Verification items for the finished model (mm, model axes). Face numbers are marked on the shaded views. A direction names the side the tool comes from. Round coordinates to 2 decimals unless told otherwise and drop trailing zeros. Loops run counter-clockwise (first coordinate to the right, second up) from the corner with the lowest first, then second, coordinate; pieces in that order, holes last. Notation, with made-up numbers: (2.5, 16) - (53.5, 16) arc R27 ccw to (53.5, 34) - close; hole circle Ø7 at (50, 45). An arc over 180 degrees is marked (long way). Use CSV: the item, a comma, the result in double quotes.
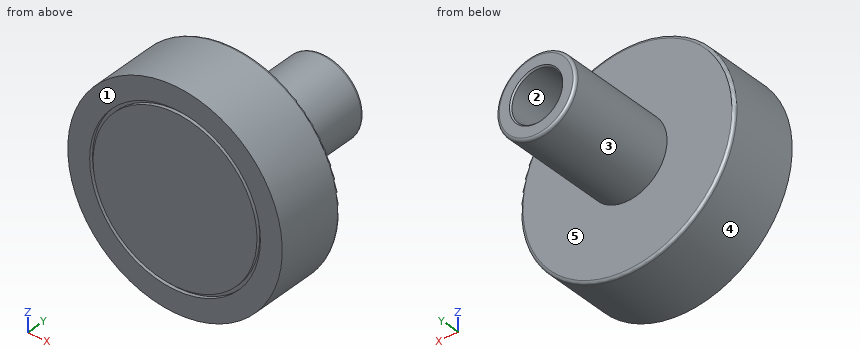
```python
from build123d import *

# Parameters (mm, degrees)
SKETCH1_R           = 7.85
BOSS_EXTRUDE1_DEPTH = 5.1
SKETCH2_R           = 2.9
BOSS_EXTRUDE2_DEPTH = 8.1
SKETCH3_R           = 1.85
CUT_EXTRUDE1_DEPTH  = 7
CHAMFER1_SIZE       = 0.1
FILLET2_R           = 0.2
SKETCH4_R           = 6.25
SKETCH4_R_2         = 6
CUT_EXTRUDE2_DEPTH  = 0.25


with BuildPart() as part:
    # Sketch1 → Boss-Extrude1 (new body)
    with BuildSketch(Plane(origin=(0, 0, 0), x_dir=(1, 0, 0), z_dir=(0, 1, 0))):
        with Locations(Location((0, 0, 0), (0, 0, 270))):
            Circle(SKETCH1_R)
    extrude(amount=-BOSS_EXTRUDE1_DEPTH)

    # Sketch2 → Boss-Extrude2 (add)
    with BuildSketch(Plane(origin=(0, 0, 0), x_dir=(1, 0, 0), z_dir=(0, 1, 0))):
        with Locations(Location((0, 0, 0), (0, 0, 270))):
            Circle(SKETCH2_R)
    extrude(amount=BOSS_EXTRUDE2_DEPTH)

    # Sketch3 → Cut-Extrude1 (cut)
    with BuildSketch(Plane(origin=(0, 8.1, 0), x_dir=(1, 0, 0), z_dir=(0, 1, 0))):
        with Locations(Location((0, 0, 0), (0, 0, 270))):
            Circle(SKETCH3_R)
    extrude(amount=-CUT_EXTRUDE1_DEPTH, mode=Mode.SUBTRACT)

    # Chamfer1
    chamfer1_edges = [part.edges().sort_by_distance(p)[0] for p in [
        (0, 8.1, -1.85),
    ]]
    chamfer(chamfer1_edges, length=CHAMFER1_SIZE)

    # Fillet2
    fillet2_edges = [part.edges().sort_by_distance(p)[0] for p in [
        (0, 0, -7.85),
        (0, 8.1, -2.9),
    ]]
    fillet(fillet2_edges, radius=FILLET2_R)

    # Sketch4 → Cut-Extrude2 (cut)
    with BuildSketch(Plane.XZ.offset(5.1)):
        with Locations(Location((0, 0, 0), (0, 0, 270))):
            Circle(SKETCH4_R)
        with Locations(Location((0, 0, 0), (0, 0, 270))):
            Circle(SKETCH4_R_2, mode=Mode.SUBTRACT)
    extrude(amount=-CUT_EXTRUDE2_DEPTH, mode=Mode.SUBTRACT)


solid = part.part
```
1) Access from +Z, -Z, +X, -X, +Y, -Y to the whole of each face (thin tool, end or side, straight path). Record for the marked faces 4 and 5.
Returned:
face 4,"+Y, -Y"
face 5,"+Y"
2) Cross-section at C-C, the plane y = 6. Record the cut outline in (x, z).
Returned:
outline,"circle Ø5.8 at (0, 0); hole circle Ø3.7 at (0, 0)"
3) Thickness scan on probe 1 along X at (y, z) = (3.75, 0); probe 2 along Y at (x, z) = (2.25, -2); probe 3 along X at (y, z) = (-3, -0.25). Record the ranges inside material, lowest first. Write a range as [from, to].
Returned:
probe 1,"x = [-2.9, -1.85], [1.85, 2.9]"
probe 2,"y = [-5.1, 0]"
probe 3,"x = [-7.85, 7.85]"
4) Cross-section at B-B, the plane z = 0. Record the cut outline in (x, y).
Returned:
outline,"(-7.85, -5.1) - (-6.25, -5.1) - (-6.25, -4.85) - (-6, -4.85) - (-6, -5.1) - (6, -5.1) - (6, -4.85) - (6.25, -4.85) - (6.25, -5.1) - (7.85, -5.1) - (7.85, -0.2) arc R0.2 ccw to (7.65, 0) - (2.9, 0) - (2.9, 7.9) arc R0.2 ccw to (2.7, 8.1) - (1.95, 8.1) - (1.85, 8) - (1.85, 1.1) - (-1.85, 1.1) - (-1.85, 8) - (-1.95, 8.1) - (-2.7, 8.1) arc R0.2 ccw to (-2.9, 7.9) - (-2.9, 0) - (-7.65, 0) arc R0.2 ccw to (-7.85, -0.2) - close"
5) Cross-section at A-A, the plane x = 0. Record the cut outline in (y, z), then the cut area to 3 significant figures.
Returned:
outline,"(-5.1, -7.85) - (-0.2, -7.85) arc R0.2 ccw to (0, -7.65) - (0, -2.9) - (7.9, -2.9) arc R0.2 ccw to (8.1, -2.7) - (8.1, -1.95) - (8, -1.85) - (1.1, -1.85) - (1.1, 1.85) - (8, 1.85) - (8.1, 1.95) - (8.1, 2.7) arc R0.2 ccw to (7.9, 2.9) - (0, 2.9) - (0, 7.65) arc R0.2 ccw to (-0.2, 7.85) - (-5.1, 7.85) - (-5.1, 6.25) - (-4.85, 6.25) - (-4.85, 6) - (-5.1, 6) - (-5.1, -6) - (-4.85, -6) - (-4.85, -6.25) - (-5.1, -6.25) - close"
area,"101 mm²"
6) Mould release check, pull along Z, two halves, no side actions. Record for the marked faces 1, 2 and 3: +Z half, -Z half, draft (parallel to the pull), parting line (faces both ways), or undercut.
Returned:
face 1,"draft"
face 2,"undercut"
face 3,"parting line"
7) Cross-section at D-D, the plane y = -3.5. Record the cut outline in (x, z), then the cut area to 3 significant figures.
Returned:
outline,"circle Ø15.7 at (0, 0)"
area,"194 mm²"
8) Gauge pin test, flat ends, axial feed: pin 1 Ø1.5 at (y, z) = (-1, 3.5) entering from +X; pin 2 Ø2 at (y, z) = (3, -4.5) entering from +X; pin 3 Ø3.5 at (x, z) = (0, 0) entering from +Y; pin 4 Ø3 at (x, y) = (4, 4) entering from -Z. Record the tip position at first contact, or that the pin passes through.
Returned:
pin 1,"stops at x = 7.35"
pin 2,"passes through"
pin 3,"stops at y = 1.1"
pin 4,"stops at z = -1.47"
